```python
from build123d import *

# Parameters (mm, degrees)
PAD001_DEPTH        = 30
HOLE002_D           = 5.5
HOLE002_CSINK_D     = 10
HOLE002_CSINK_ANGLE = 90
SKETCH004_R         = 6.501169
SKETCH004_R_2       = 5.481256
POCKET_DEPTH        = 19.5081110955
SKETCH007_W         = 3.5
SKETCH007_H         = 30
POCKET002_DEPTH     = 1
CHAMFER_SIZE        = 0.99
FILLET003_R         = 3


with BuildPart() as part:
    # Sketch002 → Pad001 (new body)
    with BuildSketch(Plane.YZ):
        with BuildLine():
            Line((-188.1964293023, 612.8903873712), (-178.5707253545, 636.394612861))
            Line((-170.2420872134, 632.9837791337), (-178.5707253545, 636.394612861))
            Line((-165.8796609268, 598.7789660675), (-170.2420872134, 632.9837791337))
            Line((-169.6694761794, 589.5249236885), (-165.8796609268, 598.7789660675))
            Line((-188.1775609373, 597.1045541936), (-169.6694761794, 589.5249236885))
            ThreePointArc((-188.1775609373, 597.1045541936), (-183.51155378, 605.0030592067), (-188.1964293023, 612.8903873712))
        make_face()
    extrude(amount=PAD001_DEPTH)

    # Hole002 (through all)
    with Locations(Plane(origin=(0, -366.8597668241, 150.2403687946), x_dir=(0, 0.3789815253, 0.9254042379), z_dir=(0, 0.9254042379, -0.3789815253))):
        with Locations((-506.967621, 13.13074), (504.2472658549, 15)):
            CounterSinkHole(HOLE002_D / 2, HOLE002_CSINK_D / 2, counter_sink_angle=HOLE002_CSINK_ANGLE)

    # Sketch004 (on DatumPlane) → Pocket (cut, through all)
    with BuildSketch(Plane(origin=(0, -366.8597668241, 150.2403687946), x_dir=(0, 0.3789815253, 0.9254042379), z_dir=(0, 0.9254042379, -0.3789815253))):
        with Locations((-506.967621, 13.13074)):
            Circle(SKETCH004_R)
        with Locations((504.2472658549, 15)):
            Circle(SKETCH004_R_2)
    extrude(amount=POCKET_DEPTH, mode=Mode.SUBTRACT)

    # Sketch007 (on Face6 of Pocket) → Pocket002 (cut)
    with BuildSketch(Plane(origin=(0, -376.1138092031, 154.0301840472), x_dir=(0, -0.3789815253, -0.9254042379), z_dir=(0, -0.9254042379, 0.3789815253))):
        with Locations((-515.7472658549, 15)):
            Rectangle(SKETCH007_W, SKETCH007_H)
    extrude(amount=-POCKET002_DEPTH, mode=Mode.SUBTRACT)

    # Chamfer
    chamfer_edges = [part.edges().sort_by_distance(p)[0] for p in [
        (15, -179.066502, 632.545365),
        (15, -180.392937, 629.306451),
    ]]
    chamfer(chamfer_edges, length=CHAMFER_SIZE)

    # Fillet003
    fillet003_edges = [part.edges().sort_by_distance(p)[0] for p in [
        (15, -188.177561, 597.104554),
        (15, -169.669476, 589.524924),
        (15, -165.879661, 598.778966),
        (15, -170.242087, 632.983779),
        (15, -178.570725, 636.394613),
        (15, -188.196429, 612.890387),
    ]]
    fillet(fillet003_edges, radius=FILLET003_R)


solid = part.part
```
Can you work these out from the model? Positions are in its coordinate system, mm. A direction names the side the tool comes from. Give positions to 0.01 mm unless a question says otherwise; leave off trailing zeros. Order: outer loops, then holes, each group sorted by start corner. A loop starts at its lowest first (then second) coordinate and runs counter-clockwise, first axis right, second up. Notation, with made-up numbers: M -7.5,18 L 38.5,18 A33 cw 38.5,55 Z; hole C -37,-7 d6. An arc over 180 degrees is marked long. One line per item, written item: value.
1) On a 3-axis mill with a long thin cutter (end or side, diameter ignored), from which of +Z, -Z, +X, -X, +Y, -Y can I reach the whole of each face in a straight line? I mean faces 1 (the face through (14.79, -167.372, 595.134)), 2 (the face through (14.79, -179.71, 632.27)). Say none if no direction works.
Answer sheet:
face 1: -Z, +X, -X, +Y
face 2: +X, -X, -Y
2) We'd pull the mould along X, two halves only. Please class faces 3 (the face through (14.79, -173.8, 634.44)), 4 (the face through (13.327, -180.651, 621.234)), 5 (the face through (13.9, -178.74, 615.24)), 6 (the face through (0, -177, 613)): released by +X, released by -X, zero draft, split by the parting line, or undercut.
Answer sheet:
face 3: zero draft
face 4: undercut
face 5: undercut
face 6: released by -X
3) I want a section at B-B, the plane z = 601. List the corners of the cut face in (x, y) for me, plus the area to 3 significant figures.
Answer sheet:
outline: M 0,-184.45 L 30,-184.45 L 30,-166.16 L 0,-166.16 Z
area: 548 mm^2
4) For P1, Ø3, axis at x = 16.5, z = 629.5, coming from the -Y side; P2, Ø5, axis at x = 15, z = 612, coming from the -Y side; P3, Ø6, axis at x = 8.5, z = 628, coming from the +Y side; P4, Ø6, axis at x = 3.5, z = 609.5, coming from the +Y side, each with a flat end and sliding along its axis, tell me the tip position at first contact or that it passes through.
Answer sheet:
P1: stops at y = -182.01
P2: stops at y = -187.52
P3: stops at y = -169.22
P4: stops at y = -166.86
5) Please list where these lines run through material, in increasing order: line 1 along X through (y, z) = (-173.5, 613.5); line 2 along X through (y, z) = (-168.75, 616); line 3 along Z through (x, y) = (15.5, -175).
Answer sheet:
line 1: x = 0 to 10.01, 19.99 to 30
line 2: x = 0 to 9.84, 20.16 to 30
line 3: z = 591.71 to 610.66, 621 to 634.93
